Check sheet for the modelled part. Datum: model origin and axes. Units: mm. A direction names the side the tool comes from. Round coordinates to 2 decimals unless told otherwise and drop trailing zeros. Write each loop counter-clockwise with the first axis right and the second up, starting at its lowest first coordinate (ties: lowest second). Pieces come first, ordered by that corner, then holes. Notation, with made-up numbers: (-28.5, 71) -> (27.5, 71) arc R6 cw to (27.5, 77) -> close; hole circle Ø10 at (66, -13.75). An arc over 180 degrees is marked (long way). One line per item, written item: value.
from build123d import *

# Parameters (mm, degrees)
F0_W     = 85.417319
F0_H     = 61.955053
F1_DEPTH = 25.4
F2_R     = 11.492787
F3_DEPTH = 12.7
F5_DEPTH = 25.4


with BuildPart() as f1:
    # F0 (on Top) → F1 (new body)
    with BuildSketch(Plane.XY):
        with Locations((5.865568, -0.641545)):
            Rectangle(F0_W, F0_H)
    extrude(amount=F1_DEPTH)

    # F2 (on face) → F3 (join)
    with BuildSketch(Plane.XY.offset(25.4)):
        with Locations((6.048867, 0)):
            Circle(F2_R)
    extrude(amount=F3_DEPTH)

    # F4 (on Front) → F5 (cut, symmetric)
    with BuildSketch(Plane.XZ):
        Polygon((18.033221, 39.003748), (-6.255646, 38.51638), (18.033221, 27.144257), align=None)
    extrude(amount=F5_DEPTH, both=True, mode=Mode.SUBTRACT)


solid = f1.part
Item 1: Sectioned sample at C-C on z = 29. Enter the section's corners in (x, y), and give its area (3 significant figures).
Answer:
outline: (14.07, -8.23) -> (14.07, 8.23) arc R11.49 ccw (long way) to start
area: 376 mm^2
Item 2: Depth check by flat-ended pin: P1, Ø4, axis at x = -12, y = -17.5, coming from the +Z side; P2, Ø5, axis at x = -1.5, y = -6, coming from the +Z side. Enter the tip coordinate at first touch or a pass-through.
Answer:
P1: stops at z = 25.4
P2: stops at z = 37.45
Item 3: Sectioned sample at B-B on x = 22. Enter the section's corners in (y, z).
Answer:
outline: (-31.62, 0) -> (30.34, 0) -> (30.34, 25.4) -> (-31.62, 25.4) -> close
Item 4: Sectioned sample at D-D on y = 19.5. Enter the section's corners in (x, z), and give its area (3 significant figures).
Answer:
outline: (-36.84, 0) -> (48.57, 0) -> (48.57, 25.4) -> (-36.84, 25.4) -> close
area: 2,170 mm^2
Item 5: Sectioned sample at A-A on y = 0. Enter the section's corners in (x, z), and give its area (3 significant figures).
Answer:
outline: (-36.84, 0) -> (48.57, 0) -> (48.57, 25.4) -> (17.54, 25.4) -> (17.54, 27.37) -> (-5.37, 38.1) -> (-5.44, 38.1) -> (-5.44, 25.4) -> (-36.84, 25.4) -> close
area: 2,340 mm^2
Item 6: Thickness scan on line 1 (Z direction, x = -13, y = -13.5); line 2 (X direction, y = -8.5, z = 27); line 3 (X direction, y = -7, z = 27). Record the ranges inside material, lowest first.
Answer:
line 1: z = 0 to 25.4
line 2: x = -1.69 to 13.78
line 3: x = -3.07 to 15.16
Item 7: Tool access check on faces 1 (the flat face through (-4, -7, 25.4)), 2 (the flat face through (5.93, -0.16, 32.81)). Record the directions out of +Z, -Z, +X, -X, +Y, -Y that give a thin tool (end or side, any length) a straight path to the whole face; none if there is none.
Answer:
face 1: +Z
face 2: +Z, +X, +Y, -Y
